Check sheet for the modelled part. Datum: model origin and axes. Units: mm. Face numbers are marked on the shaded views. A direction names the side the tool comes from. Coordinates: 2 decimals unless noted, no trailing zeros. Loops run counter-clockwise (first coordinate to the right, second up) from the corner with the lowest first, then second, coordinate; pieces in that order, holes last.
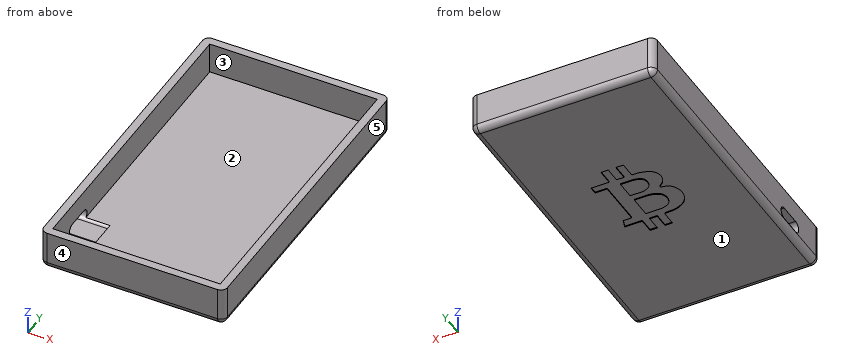
```python
from build123d import *

# Parameters (mm, degrees)
ESQUISSE1_W             = 52
ESQUISSE1_H             = 92
BOSS_EXTRU_1_DEPTH      = 9.73
COQUE1_T                = 2.5
CONG_1_R                = 2
ENL_V_MAT_EXTRU_1_DEPTH = 10
ENL_V_MAT_EXTRU_3_DEPTH = 0.3


with BuildPart() as part:
    # Esquisse1 → Boss.-Extru.1 (new body)
    with BuildSketch(Plane.XY):
        Rectangle(ESQUISSE1_W, ESQUISSE1_H)
    extrude(amount=BOSS_EXTRU_1_DEPTH)

    # Coque1
    coque1_openings = [part.faces().sort_by_distance(p)[0] for p in [
        (0, 0, 9.73),
    ]]
    offset(amount=COQUE1_T, openings=coque1_openings, kind=Kind.INTERSECTION)

    # Congé1
    # the kernel refuses this fillet: 2 mm, written as the material it takes off along each edge
    with BuildSketch(Plane(origin=(-26.5, -46.5, -0.5), x_dir=(0, 0, -1), z_dir=(-1, 0, 0))) as cong_1_piece_1_section:
        Polygon((0, 0), (CONG_1_R, 0), (CONG_1_R, CONG_1_R), (0, CONG_1_R), align=None)
    cong_1_piece_1 = extrude(amount=CONG_1_R, mode=Mode.PRIVATE)
    cong_1_piece_1 = cong_1_piece_1 - Plane(origin=(-26.5, -46.5, -0.5), x_dir=(0, 0.7071067811865475, 0.7071067811865475), z_dir=(-1, 0, 0)) * Sphere(CONG_1_R, mode=Mode.PRIVATE)
    add(cong_1_piece_1, mode=Mode.SUBTRACT)
    with BuildSketch(Plane(origin=(26.5, -46.5, -0.5), x_dir=(0, -1, 0), z_dir=(0, 0, -1))) as cong_1_piece_2_section:
        Polygon((0, 0), (CONG_1_R, 0), (CONG_1_R, -CONG_1_R), (0, -CONG_1_R), align=None)
    cong_1_piece_2 = extrude(amount=CONG_1_R, mode=Mode.PRIVATE)
    cong_1_piece_2 = cong_1_piece_2 - Plane(origin=(26.5, -46.5, -0.5), x_dir=(-0.7071067811865475, 0.7071067811865475, 0), z_dir=(0, 0, -1)) * Sphere(CONG_1_R, mode=Mode.PRIVATE)
    add(cong_1_piece_2, mode=Mode.SUBTRACT)
    with BuildSketch(Plane(origin=(-26.5, 46.5, -0.5), x_dir=(-1, 0, 0), z_dir=(0, 1, 0))) as cong_1_piece_3_section:
        Polygon((0, 0), (CONG_1_R, 0), (CONG_1_R, -CONG_1_R), (0, -CONG_1_R), align=None)
    cong_1_piece_3 = extrude(amount=CONG_1_R, mode=Mode.PRIVATE)
    cong_1_piece_3 = cong_1_piece_3 - Plane(origin=(-26.5, 46.5, -0.5), x_dir=(0.7071067811865475, 0, 0.7071067811865475), z_dir=(0, 1, 0)) * Sphere(CONG_1_R, mode=Mode.PRIVATE)
    add(cong_1_piece_3, mode=Mode.SUBTRACT)
    with BuildSketch(Plane(origin=(26.5, 46.5, -0.5), x_dir=(0, 0, -1), z_dir=(0, 1, 0))) as cong_1_piece_4_section:
        Polygon((0, 0), (CONG_1_R, 0), (CONG_1_R, -CONG_1_R), (0, -CONG_1_R), align=None)
    cong_1_piece_4 = extrude(amount=CONG_1_R, mode=Mode.PRIVATE)
    cong_1_piece_4 = cong_1_piece_4 - Plane(origin=(26.5, 46.5, -0.5), x_dir=(-0.7071067811865475, 0, 0.7071067811865475), z_dir=(0, 1, 0)) * Sphere(CONG_1_R, mode=Mode.PRIVATE)
    add(cong_1_piece_4, mode=Mode.SUBTRACT)
    with BuildSketch(Plane(origin=(-26.5, -48.5, -2.5), x_dir=(0, 0, 1), z_dir=(1, 0, 0)), Plane(origin=(26.5, 48.5, -2.5), x_dir=(0, 0, 1), z_dir=(-1, 0, 0))) as cong_1_piece_5:
        with BuildLine():
            CenterArc((CONG_1_R, -CONG_1_R), CONG_1_R, 90, 90)
            Line((0, -CONG_1_R), (0, 0))
            Line((0, 0), (CONG_1_R, 0))
        make_face()
    extrude(amount=53, mode=Mode.SUBTRACT)
    with BuildSketch(Plane(origin=(-28.5, 46.5, -2.5), x_dir=(0, 0, 1), z_dir=(0, -1, 0)), Plane(origin=(28.5, -46.5, -2.5), x_dir=(0, 0, 1), z_dir=(0, 1, 0))) as cong_1_piece_6:
        with BuildLine():
            CenterArc((CONG_1_R, -CONG_1_R), CONG_1_R, 90, 90)
            Line((0, -CONG_1_R), (0, 0))
            Line((0, 0), (CONG_1_R, 0))
        make_face()
    extrude(amount=93, mode=Mode.SUBTRACT)
    with BuildSketch(Plane(origin=(28.5, -48.5, -0.5), x_dir=(-1, 0, 0), z_dir=(0, 0, 1)), Plane(origin=(-28.5, -48.5, 14.73), x_dir=(1, 0, 0), z_dir=(0, 0, -1)), Plane(origin=(-28.5, 48.5, -0.5), x_dir=(1, 0, 0), z_dir=(0, 0, 1)), Plane(origin=(28.5, 48.5, -0.5), x_dir=(0, -1, 0), z_dir=(0, 0, 1))) as cong_1_piece_7:
        with BuildLine():
            CenterArc((CONG_1_R, -CONG_1_R), CONG_1_R, 90, 90)
            Line((0, -CONG_1_R), (0, 0))
            Line((0, 0), (CONG_1_R, 0))
        make_face()
    extrude(amount=15.23, mode=Mode.SUBTRACT)

    # Esquisse2 → Enlèv. mat.-Extru.1 (cut)
    with BuildSketch(Plane.ZY.offset(28.5)):
        with BuildLine():
            Line((3.2008816, -27.740794349), (3.2008816, -34.440794349))
            ThreePointArc((3.2008816, -34.440794349), (1.4, -36.241675948), (-0.4008816, -34.440794349))
            Line((-0.4008816, -34.440794349), (-0.4008816, -27.740794349))
            ThreePointArc((-0.4008816, -27.740794349), (1.4, -25.939912749), (3.2008816, -27.740794349))
        make_face()
    extrude(amount=-ENL_V_MAT_EXTRU_1_DEPTH, mode=Mode.SUBTRACT)

    # Esquisse3 → Enlèv. mat.-Extru.3 (cut)
    with BuildSketch(Plane(origin=(2.40458604, 5.05579629, -2.5), x_dir=(-1, 0, 0), z_dir=(0, 0, -1))):
        with BuildLine():
            ThreePointArc((4.432568846, -13.261288916), (4.216995781, -13.347231146), (4.12723276, -13.561241456))
            Line((4.12723276, -13.561241456), (4.12723276, -17.926139223))
            Line((4.12723276, -17.926139223), (1.770623661, -17.926139223))
            Line((1.770623661, -17.926139223), (1.770623661, -13.395686185))
            Line((1.770623661, -13.395686185), (-0.5550959, -13.395686185))
            Line((-0.5550959, -13.395686185), (-0.5550959, -17.926139223))
            Line((-0.5550959, -17.926139223), (-2.840872053, -17.926139223))
            Line((-2.840872053, -17.926139223), (-2.840872053, -13.395686185))
            Line((-2.840872053, -13.395686185), (-8.285917815, -13.395686185))
            Line((-8.285917815, -13.395686185), (-7.384139614, -10.715400976))
            Line((-7.384139614, -10.715400976), (-4.73260744, -10.715400976))
            Line((-4.73260744, -10.715400976), (-4.73260744, 3.629932304))
            Line((-4.73260744, 3.629932304), (-8.481683027, 3.629932304))
            Line((-8.481683027, 3.629932304), (-8.481683027, 6.035056002))
            Line((-8.481683027, 6.035056002), (-2.840872053, 6.035056002))
            Line((-2.840872053, 6.035056002), (-2.840872053, 10.899070066))
            Line((-2.840872053, 10.899070066), (-0.5550959, 10.899070066))
            Line((-0.5550959, 10.899070066), (-0.5550959, 6.035056002))
            Line((-0.5550959, 6.035056002), (1.770623661, 6.035056002))
            Line((1.770623661, 6.035056002), (1.770623661, 10.899070066))
            Line((1.770623661, 10.899070066), (4.12723276, 10.899070066))
            Line((4.12723276, 10.899070066), (4.12723276, 6.246143352))
            ThreePointArc((4.12723276, 6.246143352), (4.227791491, 6.022038064), (4.46205396, 5.948171065))
            add(Edge.make_bspline(
                [(4.432568846, -13.261288916), (4.849636806, -13.268708458), (5.98048136, -13.271449308), (7.794832478, -13.090271032), (9.783873696, -12.344515621), (11.540556036, -11.052358459), (12.564181649, -9.179795832), (12.955550354, -7.143685881), (12.593966957, -5.21310593), (11.646751192, -3.465266484), (10.232722145, -2.740195794), (9.250057043, -2.561034839), (8.750477475, -2.542580923), (8.50068383, -2.219648818), (8.784009377, -1.934125986), (9.226109387, -1.668162515), (9.919121901, -1.102236302), (10.570682868, -0.118824042), (11.103114061, 1.16921053), (11.036403439, 2.73148482), (10.346932114, 4.232154462), (9.027316851, 5.196599259), (7.619143878, 5.628972396), (6.275382284, 5.94833303), (5.214289363, 6.012654431), (4.618172733, 5.966415188), (4.46205396, 5.948171065)],
                knots=[0.009261903, 0.009261903, 0.009261903, 0.009261903, 0.047134138, 0.111411615, 0.173043756, 0.237437897, 0.304153642, 0.361015466, 0.421832084, 0.478884562, 0.534307736, 0.557824401, 0.569788977, 0.5785267, 0.586794862, 0.600583119, 0.627786372, 0.665364189, 0.706885293, 0.751518655, 0.802969516, 0.850764387, 0.894339537, 0.935725195, 0.97558798, 0.989801524, 0.989801524, 0.989801524, 0.989801524], degree=3))
        make_face()
        with BuildLine():
            Line((-0.5550959, 3.686744271), (3.348191015, 3.686744271))
            add(Edge.make_bspline(
                [(3.348191015, 3.686744271), (4.141267216, 3.56069148), (5.366493628, 3.347369666), (6.283213897, 2.246261692), (6.444658055, 1.326625386), (6.441596122, 0.427967574), (6.110231896, -0.541286606), (5.40923725, -1.183233231), (4.474914869, -1.684808073), (3.757208507, -1.861144467), (3.348191015, -1.921662594)],
                knots=[0, 0, 0, 0, 0.269919589, 0.369123458, 0.441025413, 0.567546851, 0.657930272, 0.763523098, 0.865803246, 1, 1, 1, 1], degree=3))
            Line((3.348191015, -1.921662594), (-0.5550959, -1.921662594))
            Line((-0.5550959, -1.921662594), (-0.5550959, 3.686744271))
        make_face(mode=Mode.SUBTRACT)
        with BuildLine():
            Line((-0.42913087, -4.167643381), (3.992403585, -4.167643381))
            add(Edge.make_bspline(
                [(3.992403585, -4.167643381), (4.587512864, -4.272183954), (5.572497818, -4.32153134), (6.639994555, -5.013685273), (7.566714866, -5.647143489), (8.000595426, -6.907925525), (7.999345796, -8.175630682), (7.65286389, -9.305868029), (6.888383055, -10.137129269), (5.696203316, -10.591976345), (4.820749189, -10.938794377), (4.302446939, -10.89171276)],
                knots=[0, 0, 0, 0, 0.161654957, 0.24756242, 0.333429326, 0.451191423, 0.578889109, 0.665800718, 0.756992871, 0.864854658, 1, 1, 1, 1], degree=3))
            Line((4.302446939, -10.89171276), (-0.42913087, -10.89171276))
            Line((-0.42913087, -10.89171276), (-0.42913087, -4.167643381))
        make_face(mode=Mode.SUBTRACT)
    extrude(amount=-ENL_V_MAT_EXTRU_3_DEPTH, mode=Mode.SUBTRACT)


solid = part.part
```
1) Depth check by flat-ended pin: pin 1 (10 mm diameter, centred on x = -2, y = -5, fed in from +Z). Enter the tip coordinate at first touch or a pass-through.
Answer sheet:
pin 1: stops at z = 0
2) Section check A-A on z = 8.75. Enter the section's corners in (x, y), plus the area to 3 significant figures.
Answer sheet:
outline: (-28.5, -46.5) arc R2 ccw to (-26.5, -48.5) - (26.5, -48.5) arc R2 ccw to (28.5, -46.5) - (28.5, 46.5) arc R2 ccw to (26.5, 48.5) - (-26.5, 48.5) arc R2 ccw to (-28.5, 46.5) - close; hole (-26, -46) - (26, -46) - (26, 46) - (-26, 46) - close
area: 742 mm2
3) Section check D-D on z = 1.4. Enter the section's corners in (x, y).
Answer sheet:
outline: (-28.5, -46.5) arc R2 ccw to (-26.5, -48.5) - (26.5, -48.5) arc R2 ccw to (28.5, -46.5) - (28.5, 46.5) arc R2 ccw to (26.5, 48.5) - (-26.5, 48.5) arc R2 ccw to (-28.5, 46.5) - (-28.5, -25.94) - (-26, -25.94) - (-26, 46) - (26, 46) - (26, -46) - (-26, -46) - (-26, -36.24) - (-28.5, -36.24) - close
4) Scan lines: line 1 (X direction, y = 22.5, z = 2.5); line 2 (Y direction, x = 18, z = 7.5); line 3 (Z direction, x = 6, y = -41). Record each from-to range of solid material in increasing order.
Answer sheet:
line 1: x = -28.5 to -26, 26 to 28.5
line 2: y = -48.5 to -46, 46 to 48.5
line 3: z = -2.5 to 0
5) Section check B-B on x = 17. Enter the section's corners in (y, z).
Answer sheet:
outline: (-48.5, -0.5) arc R2 ccw to (-46.5, -2.5) - (46.5, -2.5) arc R2 ccw to (48.5, -0.5) - (48.5, 9.73) - (46, 9.73) - (46, 0) - (-46, 0) - (-46, 9.73) - (-48.5, 9.73) - close
6) Mould release check, pull along X, two halves, no side actions. Record for the marked faces 3, 4 and 5: +X half, -X half, draft (parallel to the pull), parting line (faces both ways), or undercut.
Answer sheet:
face 3: undercut
face 4: draft
face 5: +X half
7) Set-up check for the marked faces 1 and 2: record each of +Z, -Z, +X, -X, +Y, -Y from which the full face is reachable in a straight line by a thin tool's end or side.
Answer sheet:
face 1: -Z, +X, -X, +Y, -Y
face 2: +Z
8) Section check C-C on y = 23. Enter the section's corners in (x, z).
Answer sheet:
outline: (-28.5, -0.5) arc R2 ccw to (-26.5, -2.5) - (26.5, -2.5) arc R2 ccw to (28.5, -0.5) - (28.5, 9.73) - (26, 9.73) - (26, 0) - (-26, 0) - (-26, 9.73) - (-28.5, 9.73) - close
